Could you check a few things on this model? Use its own coordinates, in mm. Face numbers are marked on the shaded views. A direction names the side the tool comes from. Round coordinates to 2 decimals unless told otherwise and drop trailing zeros. Write each loop counter-clockwise with the first axis right and the second up, starting at its lowest first coordinate (ties: lowest second). Pieces come first, ordered by that corner, then holes. Notation, with made-up numbers: (47, -23.75) -> (92, -23.75) arc R10 ccw to (92, -5.75) -> close; hole circle Ø7 at (25, -28). An arc over 180 degrees is marked (long way). Return JSON: item names as keys, results as strings.
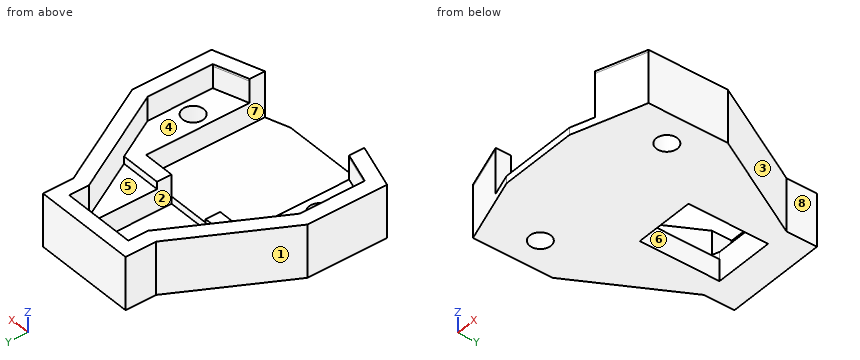
Autodesk Inventor part; units mm, degrees
ref_plane "YZ Plane" through (0, 0, 0) normal (1, 0, 0) x (0, 1, 0)
ref_plane "XZ Plane" through (0, 0, 0) normal (0, 1, 0) x (-1, 0, 0)
ref_plane "XY Plane" through (0, 0, 0) normal (0, 0, 1) x (1, 0, 0)
sketch "Sketch1" plane through (0, 0, 0) normal (0, 0, 1) x (1, 0, 0)
  line L0 (-5, -2.5) -> (5, -2.5) construction
  line L1 (5, -2.5) -> (12.675, 0) construction
  line L2 (-5, -2.5) -> (-12.675, 0)
  line L3 (12.675, 0) -> (-12.675, 0) construction
  line L4 (12.675, 0) -> (12.675, 8.7) construction
  line L5 (-12.675, 0) -> (-12.675, 8.7)
  line L6 (-12.675, 8.7) -> (-4.75, 23.2)
  line L7 (-4.75, 23.2) -> (-4.75, 25.7)
  line L8 (-4.75, 25.7) -> (4.75, 25.7) construction
  line L9 (4.75, 25.7) -> (4.75, 23.2) construction
  line L10 (4.75, 23.2) -> (12.675, 8.7) construction
  line L11 (0, -8.56) -> (0, 31.76)
  line L12 (0, 25.7) -> (0, -2.5)
  circle A0 centre (-10.8, 4.25) radius 1.25
  line L13 (-10.8, 4.25) -> (0, 4.25) construction
  line L14 (-4.75, 25.7) -> (0, 25.7)
  line L15 (-5, -2.5) -> (0, -2.5)
  line L16 (-5.05, 23.2766) -> (-12.975, 8.7766)
  line L17 (-12.975, 8.7766) -> (-12.975, -0.2178)
  line L18 (-12.975, -0.2178) -> (-5.0476, -2.8)
  line L19 (-5.0476, -2.8) -> (0.3, -2.8) construction
  line L20 (0.3, -2.8) -> (0.3, 26) construction
  line L21 (0.3, 26) -> (-5.05, 26) construction
  line L22 (-5.05, 26) -> (-5.05, 23.2766)
  line L23 (0, -2.5) -> (0, -2.8)
  line L24 (0, 25.7) -> (0, 26)
  line L25 (0, -2.8) -> (-5.0476, -2.8)
  line L26 (0, 26) -> (-5.05, 26)
  point P0 (0, 0)
  point P1 (0, 0)
  dimension "d0" = 10
  dimension "d1" = 25.35
  dimension "d2" = 2.5
  dimension "d3" = 8.7
  dimension "d4" = 28.2
  dimension "d6" = 2.5
  dimension "d7" = 9.5
  dimension "d42" = 2.5
  dimension "d43" = 10.8
  dimension "d44" = 6.75
  dimension "d53" = 0.3
sketch "Sketch8" plane through (0, 0, 0) normal (0, 0, 1) x (1, 0, 0)
  line L0 (-20, 30) -> (20, 30)
  line L1 (20, 30) -> (20, -10)
  line L2 (20, -10) -> (-20, -10)
  line L3 (-20, -10) -> (-20, 30)
  point P0 (0, 0)
  point P1 (0, -10)
  dimension "d45" = 40
  dimension "d46" = 10
extrude "MainBlock" add sketch "Sketch8" against normal blind 7
extrude "CartridgeCutout" cut sketch "Sketch1" against normal blind 3
sketch "Sketch10" plane through (-10.8, 4.25, 0) normal (0, 0, 1) x (1, 0, 0)
  circle A0 centre (0, 0) radius 1.25
  circle A1 centre (0, 0) radius 1.45
  point P0 (10.8, -4.25)
  dimension "d56" = 0.2
extrude "PinHole" cut sketch "Sketch10" against normal through all contours A0 | A1
mirror "Mirror3" about plane through (0, 26, 0) normal (-1, 0, 0) of "CartridgeCutout", "PinHole"
sketch "Sketch12" plane through (0, 0, -3) normal (0, 0, 1) x (1, 0, 0)
  circle A0 centre (10.8, 4.25) radius 1.45
  circle A1 centre (-10.8, 4.25) radius 1.45
  line L0 (5.05, 26) -> (-5.05, 26)
  line L1 (-5.05, 23.2766) -> (-5.05, 26)
  line L2 (-12.975, 8.7766) -> (-5.05, 23.2766)
  line L3 (-12.975, -0.2178) -> (-12.975, 8.7766)
  line L4 (-5.0476, -2.8) -> (-12.975, -0.2178)
  line L5 (5.0476, -2.8) -> (-5.0476, -2.8)
  line L6 (5.0476, -2.8) -> (12.975, -0.2178)
  line L7 (12.975, -0.2178) -> (12.975, 8.7766)
  line L8 (12.975, 8.7766) -> (5.05, 23.2766)
  line L9 (5.05, 23.2766) -> (5.05, 26)
  line L10 (-4.15, 23.6) -> (4.15, 23.6)
  line L11 (4.15, 23.6) -> (4.15, -1.4)
  line L12 (4.15, -1.4) -> (-4.15, -1.4)
  line L13 (-4.15, -1.4) -> (-4.15, 23.6)
  point P0 (0, 0)
  point P1 (0, -1.4)
  dimension "d59" = 8.3
  dimension "d60" = 25
  dimension "d61" = 1.4
extrude "CentreHole" cut sketch "Sketch12" against normal through all contours L10 L11 L12 L13
sketch "Sketch13" plane through (0, 0, 0) normal (0, 0, 1) x (1, 0, 0)
  line L0 (-5.05, 26) -> (5.05, 26)
  line L1 (5.05, 26) -> (5.05, 23.2766)
  line L2 (5.05, 23.2766) -> (12.975, 8.7766)
  line L3 (12.975, 8.7766) -> (12.975, -0.2178)
  line L4 (12.975, -0.2178) -> (5.0476, -2.8)
  line L5 (5.0476, -2.8) -> (-5.0476, -2.8)
  line L6 (-5.0476, -2.8) -> (-12.975, -0.2178)
  line L7 (-12.975, -0.2178) -> (-12.975, 8.7766)
  line L8 (-12.975, 8.7766) -> (-5.05, 23.2766)
  line L9 (-5.05, 23.2766) -> (-5.05, 26)
  line L10 (-20, 30) -> (20, 30)
  line L11 (-20, -10) -> (-20, 30)
  line L12 (20, -10) -> (-20, -10)
  line L13 (20, 30) -> (20, -10)
  line L14 (-14.975, 9.2875) -> (-14.975, -1.6698)
  line L15 (-14.975, -1.6698) -> (-5.3652, -4.8)
  line L16 (-5.3652, -4.8) -> (5.3652, -4.8)
  line L17 (5.3652, -4.8) -> (14.975, -1.6698)
  line L18 (14.975, -1.6698) -> (14.975, 9.2875)
  line L19 (14.975, 9.2875) -> (7.05, 23.7875)
  line L20 (7.05, 23.7875) -> (7.05, 28)
  line L21 (7.05, 28) -> (-7.05, 28)
  line L22 (-7.05, 28) -> (-7.05, 23.7875)
  line L23 (-7.05, 23.7875) -> (-14.975, 9.2875)
  point P0 (0, 0)
  dimension "d65" = 2
extrude "OutlineCut" cut sketch "Sketch13" against normal through all contours L10 L13 L12 L11
sketch "Sketch14" plane through (0, 0, -3) normal (0, 0, 1) x (1, 0, 0)
  line L0 (-4.15, -1.4) -> (-4.15, 23.6)
  line L1 (-4.15, 23.6) -> (4.15, 23.6)
  line L2 (4.15, 23.6) -> (4.15, -1.4)
  line L3 (4.15, -1.4) -> (-4.15, -1.4) construction
  circle A0 centre (10.8, 4.25) radius 1.45 construction
  circle A1 centre (-10.8, 4.25) radius 1.45 construction
  line L4 (5.05, 26) -> (-5.05, 26)
  line L5 (-5.05, 23.2766) -> (-5.05, 26)
  line L6 (-12.975, 8.7766) -> (-5.05, 23.2766)
  line L7 (-12.975, -0.2178) -> (-12.975, 8.7766) construction
  line L8 (-5.0476, -2.8) -> (-12.975, -0.2178) construction
  line L9 (5.0476, -2.8) -> (-5.0476, -2.8) construction
  line L10 (5.0476, -2.8) -> (12.975, -0.2178) construction
  line L11 (12.975, -0.2178) -> (12.975, 8.7766) construction
  line L12 (12.975, 8.7766) -> (5.05, 23.2766)
  line L13 (5.05, 23.2766) -> (5.05, 26)
  line L14 (-9.7922, 14.6) -> (-4.15, 14.6)
  line L15 (-12.975, 8.7766) -> (-5.05, 23.2766)
  line L16 (-4.15, 23.6) -> (-5.05, 23.2766)
  line L17 (0, -18) -> (0, 38)
  line L18 (-4.15, 23.6) -> (-4.15, 14.6)
  line L19 (-4.15, -1.4) -> (-4.15, 23.6)
  line L20 (-5.05, 23.2766) -> (-9.7922, 14.6)
  line L21 (-12.975, 8.7766) -> (-5.05, 23.2766)
  line L22 (9.7922, 14.6) -> (4.15, 14.6)
  line L23 (4.15, 23.6) -> (5.05, 23.2766)
  line L24 (4.15, 23.6) -> (4.15, 14.6)
  line L25 (5.05, 23.2766) -> (9.7922, 14.6)
  point P0 (0, 0)
  dimension "d70" = 9
extrude "AlignmentGooveCut" cut sketch "Sketch14" against normal blind 1 contours L14 L6 L16 L0 | L23 L12 L22 L2
sketch "Sketch16" plane through (0, 0, 0) normal (0, 0, 1) x (1, 0, 0)
  line L0 (-8.5, 12.6) -> (8.5, 12.6)
  line L1 (8.5, 12.6) -> (8.5, -7.4)
  line L2 (8.5, -7.4) -> (-8.5, -7.4)
  line L3 (-8.5, -7.4) -> (-8.5, 12.6)
  line L4 (4.15, -1.4) -> (-4.15, -1.4)
  point P0 (0, 0)
  point P1 (0, -7.4)
  dimension "d73" = 17
  dimension "d74" = 20
  dimension "d75" = 14
extrude "CircuitBoardCut" cut sketch "Sketch16" against normal blind 6
sketch "Sketch18" plane through (0, 0, -6) normal (0, 0, 1) x (1, 0, 0)
  line L0 (-4.15, 12.6) -> (-4.15, -1.4)
  line L1 (-4.15, -1.4) -> (4.15, -1.4)
  line L2 (4.15, -1.4) -> (4.15, 12.6)
  line L3 (-4.15, 12.6) -> (4.15, 12.6)
  line L4 (-4.15, 23.6) -> (-4.15, -1.4)
  point P0 (0, 0)
extrude "CircuitBoardFillIn" add sketch "Sketch18" against normal up to surface (1 mm away)
sketch "Sketch19" plane through (0, 0, 0) normal (0, 0, 1) x (1, 0, 0)
  line L0 (8.5, -1.6754) -> (8.5, -3.7789)
  line L1 (8.5, -3.7789) -> (14.975, -1.6698)
  line L2 (14.975, -1.6698) -> (14.975, 9.2875)
  line L3 (14.975, 9.2875) -> (7.05, 23.7875)
  line L4 (7.05, 23.7875) -> (7.05, 28)
  line L5 (-7.05, 28) -> (-7.05, 23.7875)
  line L6 (-7.05, 23.7875) -> (-14.975, 9.2875)
  line L7 (-14.975, 9.2875) -> (-14.975, -1.6698)
  line L8 (-14.975, -1.6698) -> (-8.5, -3.7789)
  line L9 (-8.5, -3.7789) -> (-8.5, -1.6754)
  line L10 (-8.5, -1.6754) -> (-12.975, -0.2178)
  line L11 (-12.975, -0.2178) -> (-12.975, 8.7766)
  line L12 (-12.975, 8.7766) -> (-5.05, 23.2766)
  line L13 (-5.05, 23.2766) -> (-5.05, 26)
  line L14 (-5.05, 26) -> (5.05, 26)
  line L15 (5.05, 26) -> (5.05, 23.2766)
  line L16 (5.05, 23.2766) -> (12.975, 8.7766)
  line L17 (12.975, 8.7766) -> (12.975, -0.2178)
  line L18 (12.975, -0.2178) -> (8.5, -1.6754)
  line L19 (7.05, 28) -> (-7.05, 28)
  point P0 (0, 0)
extrude "TopHeightAdjustment" add sketch "Sketch19" along normal blind 0.3
properties part number "InkjetHolderV5"
1) For the marked faces 5, 6, 7 and 8, which set-ups out of +Z, -Z, +X, -X, +Y, -Y let a thin tool reach every point of the face, with its end or its side?
Return value:
{"face 5": "+Z", "face 6": "+Z, -Z", "face 7": "+Z, -Y", "face 8": "+Z, -Z, +X, +Y"}
2) Thinking about a two-plate mould opening in X: for the marked faces 1, 2, 3 and 4, which applies, pulls with the +X half, pulls with the -X half, needs draft (parallel to the pull), parting line crosses it, or undercut?
Return value:
{"face 1": "pulls with the -X half", "face 2": "undercut", "face 3": "pulls with the +X half", "face 4": "undercut"}
3) I want a section at D-D, the plane y = 13. Please give me the cut outline in (x, z), and give its area (3 significant figures).
Return value:
{"outline": "(-12.95, -7) -> (-4.15, -7) -> (-4.15, -3) -> (-10.67, -3) -> (-10.67, 0.3) -> (-12.95, 0.3) -> close; (4.15, -7) -> (12.95, -7) -> (12.95, 0.3) -> (10.67, 0.3) -> (10.67, -3) -> (4.15, -3) -> close", "area": "85.4 mm²"}
4) Will these pins go through, and if not, where does the flat tip stop? pin 1 Ø1.5 at (x, z) = (-5.5, -4) entering from -Y; pin 2 Ø3.5 at (y, z) = (25, -2) entering from +X; pin 3 Ø7 at (x, y) = (8, 9.5) entering from +Z.
Return value:
{"pin 1": "y = 12.6", "pin 2": "x = 7.34", "pin 3": "z = -3"}
5) I want a section at B-B, the plane z = -3.5. Count the separate pieces of the cut face and the enclosed holes in it, and give its area (3 significant figures).
Return value:
{"separate pieces": "1", "enclosed holes": "2", "area": "316 mm²"}
6) If I drill on probe 1 along X at (y, z) = (4, -2.5) (3 decimals); probe 2 along Z at (x, y) = (-1, 10); probe 3 along Y at (x, z) = (-1.25, -3.5), over which ranges is the centre line in solid material (lowest first)? Write a range as [from, to].
Return value:
{"probe 1": "[-14.975, -12.975], [12.975, 14.975]", "probe 2": "[-7, -6]", "probe 3": "[23.6, 28]"}
7) I want a section at A-A, the plane y = 4.25. Please give me the cut outline in (x, z) (3 decimals).
Return value:
{"outline": "(-14.975, -7) -> (-12.25, -7) -> (-12.25, -3) -> (-12.975, -3) -> (-12.975, 0.3) -> (-14.975, 0.3) -> close; (-9.35, -7) -> (9.35, -7) -> (9.35, -3) -> (8.5, -3) -> (8.5, -6) -> (-8.5, -6) -> (-8.5, -3) -> (-9.35, -3) -> close; (12.25, -7) -> (14.975, -7) -> (14.975, 0.3) -> (12.975, 0.3) -> (12.975, -3) -> (12.25, -3) -> close"}
8) I want a section at C-C, the plane x = 2.75. Please give me the cut outline in (y, z).
Return value:
{"outline": "(-4.8, -7) -> (12.6, -7) -> (12.6, -6) -> (-4.8, -6) -> close; (23.6, -7) -> (28, -7) -> (28, 0.3) -> (26, 0.3) -> (26, -3) -> (23.6, -3) -> close"}
